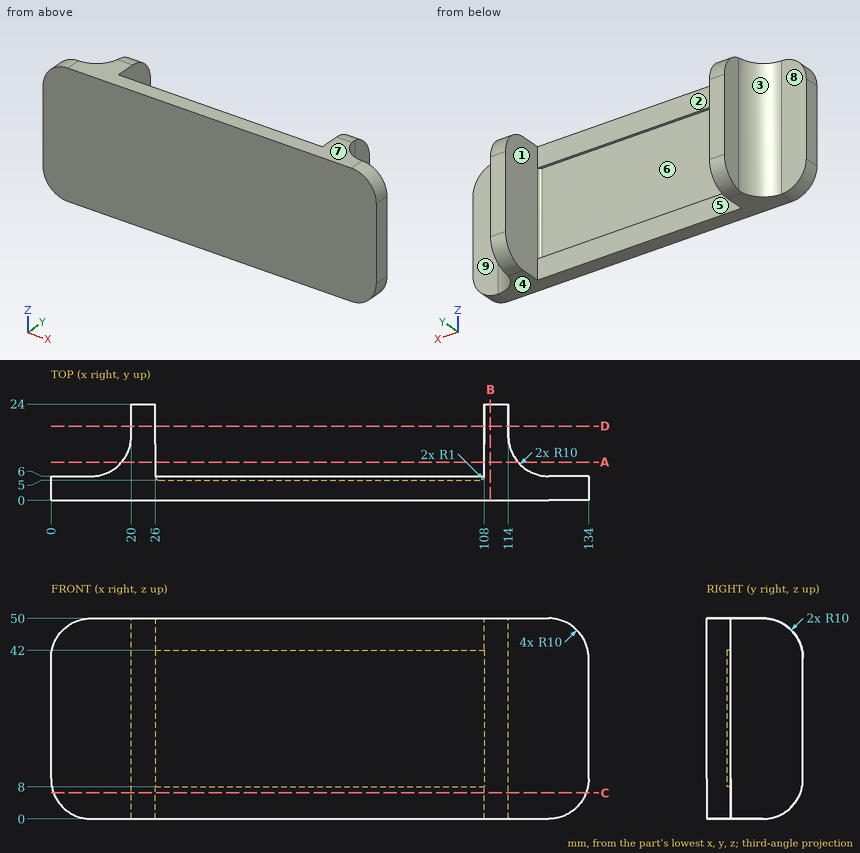
Source: three-view drawing plus pictorial views. Frame: mm from the lowest corner of the part. A direction names the side the tool comes from. Round coordinates to 2 decimals unless told otherwise and drop trailing zeros. Write each loop counter-clockwise with the first axis right and the second up, starting at its lowest first coordinate (ties: lowest second). Pieces come first, ordered by that corner, then holes. Notation, with made-up numbers: (-31.75, 70.25) -> (5.25, 70.25) arc R23 cw to (5.25, 106.25) -> close; hole circle Ø2 at (42, -30). An arc over 180 degrees is marked (long way). Return JSON: item names as keys, results as strings.
Q1. Section D-D on y = 18.5. Return the cut outline in (x, z), and give its area (3 significant figures).
From the geometry:
{"outline": "(20, 1.07) -> (26, 1.07) -> (26, 48.93) -> (20, 48.93) -> close; (108, 1.07) -> (114, 1.07) -> (114, 48.93) -> (108, 48.93) -> close", "area": "574 mm2"}
Q2. Section A-A on y = 9.5. Return the cut outline in (x, z).
From the geometry:
{"outline": "(17.6, 0) -> (26, 0) -> (26, 50) -> (17.6, 50) -> close; (108, 0) -> (116.4, 0) -> (116.4, 50) -> (108, 50) -> close"}
Q3. First-contact query: pin 1 Ø3 at (x, z) = (131, 30.5) entering from +Y; pin 2 Ø1 at (y, z) = (14, 15.5) entering from +X; pin 3 Ø2.5 at (y, z) = (19, 30) entering from +X. Flat tips, straight axial feed; report the tip coordinate or a pass-through.
From the geometry:
{"pin 1": "y = 6", "pin 2": "x = 114.32", "pin 3": "x = 114"}
Q4. Set-up query: the marked faces 5, 6, 7, 8 and 9. Return all of +Z, -Z, +X, -X, +Y, -Y with unobstructed straight access to the full face (end or side cutting, diameter ignored); none if empty.
From the geometry:
{"face 5": "+Z, -Z, +Y", "face 6": "+Y", "face 7": "+Z, +X, -X, +Y, -Y", "face 8": "+Z, -Z, -X, +Y", "face 9": "+Z, -Z, +X, +Y"}
Q5. Section B-B on x = 109.5. Return the cut outline in (y, z).
From the geometry:
{"outline": "(0, 0) -> (14, 0) arc R10 ccw to (24, 10) -> (24, 40) arc R10 ccw to (14, 50) -> (0, 50) -> close"}
Q6. Ray query, line 1 (X direction, y = 19, z = 37.5); line 2 (Y direction, x = 72.5, z = 27); line 3 (Y direction, x = 47.5, z = 43). Return the intervals inside material, ascending.
From the geometry:
{"line 1": "20 to 26, 108 to 114", "line 2": "0 to 5", "line 3": "0 to 6"}
Q7. Section C-C on z = 6.5. Return the cut outline in (x, y), and give its area (3 significant figures).
From the geometry:
{"outline": "(0.63, 0) -> (133.37, 0) -> (133.37, 6) -> (124, 6) arc R10 cw to (114, 16) -> (114, 23.37) -> (108, 23.37) -> (108, 6) -> (26, 6) -> (26, 23.37) -> (20, 23.37) -> (20, 16) arc R10 cw to (10, 6) -> (0.63, 6) -> close", "area": "1,050 mm2"}
Q8. Mould query, pull axis X, two halves, no side actions, for the marked faces 1, 2, 3 and 4. Classes: +X half, -X half, draft (parallel to the pull), parting line (faces both ways), or undercut.
From the geometry:
{"face 1": "undercut", "face 2": "undercut", "face 3": "-X half", "face 4": "draft"}
